Check sheet for the drawn part. Datum: minimum x, y, z corner. Units: mm. A direction names the side the tool comes from. Coordinates: 2 decimals unless noted, no trailing zeros. Loops run counter-clockwise (first coordinate to the right, second up) from the corner with the lowest first, then second, coordinate; pieces in that order, holes last.
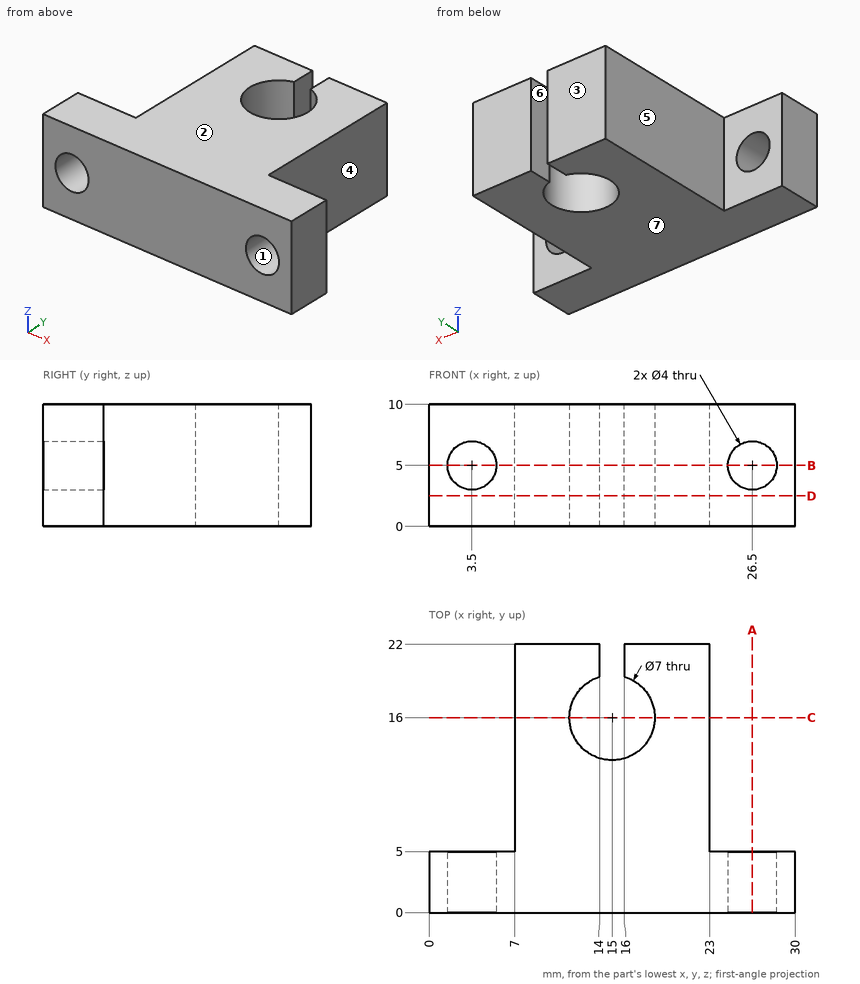
(1) Sectioned sample at D-D on z = 2.5. Record the cut outline in (x, y), and give its area (3 significant figures).
Findings:
outline: (0, 0) - (30, 0) - (30, 5) - (23, 5) - (23, 22) - (16, 22) - (16, 19.35) arc R3.5 cw (long way) to (14, 19.35) - (14, 22) - (7, 22) - (7, 5) - (0, 5) - close
area: 378 mm2
(2) Gauge pin test, flat ends, axial feed: pin 1 Ø1 at (y, z) = (15, 4) entering from -X; pin 2 Ø3 at (y, z) = (13.5, 4) entering from +X; pin 3 Ø12 at (x, y) = (24, 19) entering from +Z; pin 4 Ø5.5 at (x, z) = (26.5, 4) entering from +Y. Record the tip position at first contact, or that the pin passes through.
Findings:
pin 1: stops at x = 7
pin 2: stops at x = 23
pin 3: stops at z = 10
pin 4: stops at y = 5
(3) Sectioned sample at B-B on z = 5. Record the cut outline in (x, y), and give its area (3 significant figures).
Findings:
outline: (0, 0) - (1.5, 0) - (1.5, 5) - (0, 5) - close; (5.5, 0) - (24.5, 0) - (24.5, 5) - (23, 5) - (23, 22) - (16, 22) - (16, 19.35) arc R3.5 cw (long way) to (14, 19.35) - (14, 22) - (7, 22) - (7, 5) - (5.5, 5) - close; (28.5, 0) - (30, 0) - (30, 5) - (28.5, 5) - close
area: 338 mm2
(4) Sectioned sample at C-C on y = 16. Record the cut outline in (x, z).
Findings:
outline: (7, 0) - (11.5, 0) - (11.5, 10) - (7, 10) - close; (18.5, 0) - (23, 0) - (23, 10) - (18.5, 10) - close
(5) Access from +Z, -Z, +X, -X, +Y, -Y to the whole of each face (thin tool, end or side, straight path). Record for the marked faces 4, 5, 6 and 7.
Findings:
face 4: +Z, -Z, +X, +Y
face 5: +Z, -Z, -X, +Y
face 6: +Z, -Z, +Y
face 7: -Z, +X, -X, +Y, -Y
(6) Draft check along Z on the marked faces 1, 2 and 3. Enter one of: +Z half, -Z half, draft (parallel to the pull), parting line (faces both ways), or undercut.
Findings:
face 1: undercut
face 2: +Z half
face 3: draft
(7) Scan lines: L1, parallel to X at y = 16, z = 3.5; L2, parallel to X at y = 20.5, z = 7; L3, parallel to Z at x = 26.5, y = 2.4. Record each from-to range of solid material in increasing order.
Findings:
L1: x = 7 to 11.5, 18.5 to 23
L2: x = 7 to 14, 16 to 23
L3: z = 0 to 3, 7 to 10
(8) Sectioned sample at A-A on x = 26.5. Record the cut outline in (y, z), and give its area (3 significant figures).
Findings:
outline: (0, 0) - (5, 0) - (5, 3) - (0, 3) - close; (0, 7) - (5, 7) - (5, 10) - (0, 10) - close
area: 30.0 mm2
